Build history of the part. All positions in model axes, mm. Face numbers are marked on the shaded views. A direction names the side the tool comes from. Give positions to 0.01 mm unless a question says otherwise; leave off trailing zeros. Order: outer loops, then holes, each group sorted by start corner. A loop starts at its lowest first (then second) coordinate and runs counter-clockwise, first axis right, second up. Notation, with made-up numbers: M 76.25,1 L 83.25,1 A13 ccw 83.25,11 Z; hole C 74,-27.5 d10. An arc over 180 degrees is marked long. Answer as CSV lines item,"result".
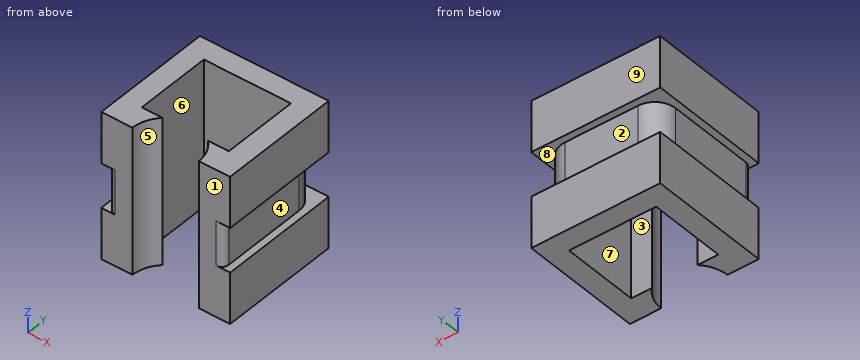
from build123d import *

# Parameters (mm, degrees)
BOSS_EXTRUDE1_DEPTH = 10.5
CUT_EXTRUDE1_DEPTH  = 3.175
FILLET1_R           = 3
FILLET2_R           = 1


with BuildPart() as part:
    # Sketch1 → Boss-Extrude1 (new, symmetric)
    with BuildSketch(Plane.XY):
        with BuildLine():
            Line((-4.7625, 0), (-9.25, 0))
            Line((-9.25, 0), (-9.25, 17.5125))
            Line((-9.25, 17.5125), (9.25, 17.5125))
            Line((9.25, 17.5125), (9.25, 0))
            Line((9.25, 0), (4.7625, 0))
            ThreePointArc((4.7625, 0), (4.368039105, 1.89779889), (3.25, 3.481221948))
            Line((3.25, 3.481221948), (6.25, 3.481221948))
            Line((6.25, 3.481221948), (6.25, 14.5125))
            Line((6.25, 14.5125), (-6.25, 14.5125))
            Line((-6.25, 14.5125), (-6.25, 3.481221948))
            Line((-6.25, 3.481221948), (-3.25, 3.481221948))
            ThreePointArc((-3.25, 3.481221948), (-4.368039105, 1.89779889), (-4.7625, 0))
        make_face()
    extrude(amount=BOSS_EXTRUDE1_DEPTH, both=True)

    # Sketch2 → Cut-Extrude1 (cut, symmetric)
    with BuildSketch(Plane.XY):
        Polygon((0, 17.5125), (-9.25, 17.5125), (-9.25, 0), (-8.25, 0), (-8.25, 16.5125), (0, 16.5125), align=None)
    cut_extrude1 = extrude(amount=CUT_EXTRUDE1_DEPTH, both=True, mode=Mode.SUBTRACT)

    # Mirror1: Cut-Extrude1 across plane
    add(cut_extrude1.mirror(Plane(origin=(0, 0, 0), x_dir=(0, 0, 1), z_dir=(1, 0, 0))), mode=Mode.SUBTRACT)

    # Fillet1
    fillet1_edges = [part.edges().sort_by_distance(p)[0] for p in [
        (-8.25, 16.5125, 0),
        (8.25, 16.5125, 0),
    ]]
    fillet(fillet1_edges, radius=FILLET1_R)

    # Fillet2
    fillet2_edges = [part.edges().sort_by_distance(p)[0] for p in [
        (-8.25, 0, 0),
        (8.25, 0, 0),
    ]]
    fillet(fillet2_edges, radius=FILLET2_R)


solid = part.part
Item 1: Drop flat-ended pins along their axis: pin 1 (1.5 mm diameter, centred on x = -1, z = -2, fed in from -Y); pin 2 (5 mm diameter, centred on x = 1, z = 0.5, fed in from +Y). Give the stop position or say it passes through.
Geometry says:
pin 1,"stops at y = 14.51"
pin 2,"stops at y = 16.51"
Item 2: 3-axis set-ups, long thin cutter, end or side, ignore diameter. For the marked faces 1, 2, 3, 4 and 5: which of +Z, -Z, +X, -X, +Y, -Y reach the whole face in a straight line?
Geometry says:
face 1,"+Z, -Z, +X, -X, -Y"
face 2,"+X, -X, +Y"
face 3,"+Z, -Z"
face 4,"+X, +Y, -Y"
face 5,"+Z, -Z, -Y"
Item 3: Band-saw the part on A-A (y = 12.75). Give the cut face in (x, z) (3 decimals), and give its area (3 significant figures).
Geometry says:
outline,"M -9.25,-10.5 L -6.25,-10.5 L -6.25,10.5 L -9.25,10.5 L -9.25,3.175 L -8.25,3.175 L -8.25,-3.175 L -9.25,-3.175 Z; M 6.25,-10.5 L 9.25,-10.5 L 9.25,-3.175 L 8.25,-3.175 L 8.25,3.175 L 9.25,3.175 L 9.25,10.5 L 6.25,10.5 Z"
area,"113 mm2"
Item 4: Probe line 1 along X through (y, z) = (4, -4.25); line 2 along Y through (x, z) = (-5.75, 3.25); line 3 along X through (y, z) = (4.25, 2.75). List the from-to ranges inside material, lowest first. Write a range as from..to.
Geometry says:
line 1,"x = -9.25..-6.25, 6.25..9.25"
line 2,"y = 0..3.48, 14.51..17.51"
line 3,"x = -8.25..-6.25, 6.25..8.25"
Item 5: Band-saw the part on D-D (y = 1.5). Give the cut face in (x, z) (3 decimals).
Geometry says:
outline,"M -9.25,-10.5 L -4.52,-10.5 L -4.52,10.5 L -9.25,10.5 L -9.25,3.175 L -8.25,3.175 L -8.25,-3.175 L -9.25,-3.175 Z; M 4.52,-10.5 L 9.25,-10.5 L 9.25,-3.175 L 8.25,-3.175 L 8.25,3.175 L 9.25,3.175 L 9.25,10.5 L 4.52,10.5 Z"
Item 6: Band-saw the part on B-B (x = -2.75). Give the cut face in (y, z) (1 decimal), and give its area (4 significant figures).
Geometry says:
outline,"M 14.5,-10.5 L 17.5,-10.5 L 17.5,-3.2 L 16.5,-3.2 L 16.5,3.2 L 17.5,3.2 L 17.5,10.5 L 14.5,10.5 Z"
area,"56.65 mm2"
Item 7: Pull direction Y, two halves, no side cores. Call the marked faces 6, 7, 8 and 9: released by +Y, released by -Y, zero draft, split by the parting line, or undercut.
Geometry says:
face 6,"undercut"
face 7,"undercut"
face 8,"zero draft"
face 9,"released by +Y"
